Drawing for the job (mm, zero at the part's lowest x, y, z). Coordinates: 2 decimals unless noted, no trailing zeros. Write each loop counter-clockwise with the first axis right and the second up, starting at its lowest first coordinate (ties: lowest second). Pieces come first, ordered by that corner, then holes. Notation, with made-up numbers: M 55.5,32.5 L 112.5,32.5 A21 cw 112.5,37.5 Z; hole C -8,15 d7. An arc over 180 degrees is marked long. Put each result on its own line as item: value. Start each with the question number.
Q1. Cut at D-D (x = 14.75). Write the cut outline in (y, z), then the cut area to 3 significant figures.
Q2. Drill centre lines: line 1 along X through (y, z) = (2.75, 6.5); line 2 along X through (y, z) = (6.5, 6.5); line 3 along X through (y, z) = (4.75, 6.75). Where is each one in solid material? Low to high.
Q3. Cut at C-C (y = 5.25). Write the cut outline in (x, z).
Q4. Pull direction Z, two halves, no side cores. Call the marked faces 1, 2, 3 and 4: pulls with the +Z half, pulls with the -Z half, needs draft (parallel to the pull), parting line crosses it, or undercut.
Q5. Cut at B-B (z = 6.5). Write the cut outline in (x, y).
Q6. Cut at A-A (y = 7). Write the cut outline in (x, z).
Q7. Drop flat-ended pins along their axis: pin 1 (2 mm diameter, centred on y = 4, z = 11.5, fed in from +X); pin 2 (1.5 mm diameter, centred on y = 5.5, z = 10, fed in from -X). Give the stop position or say it passes through.
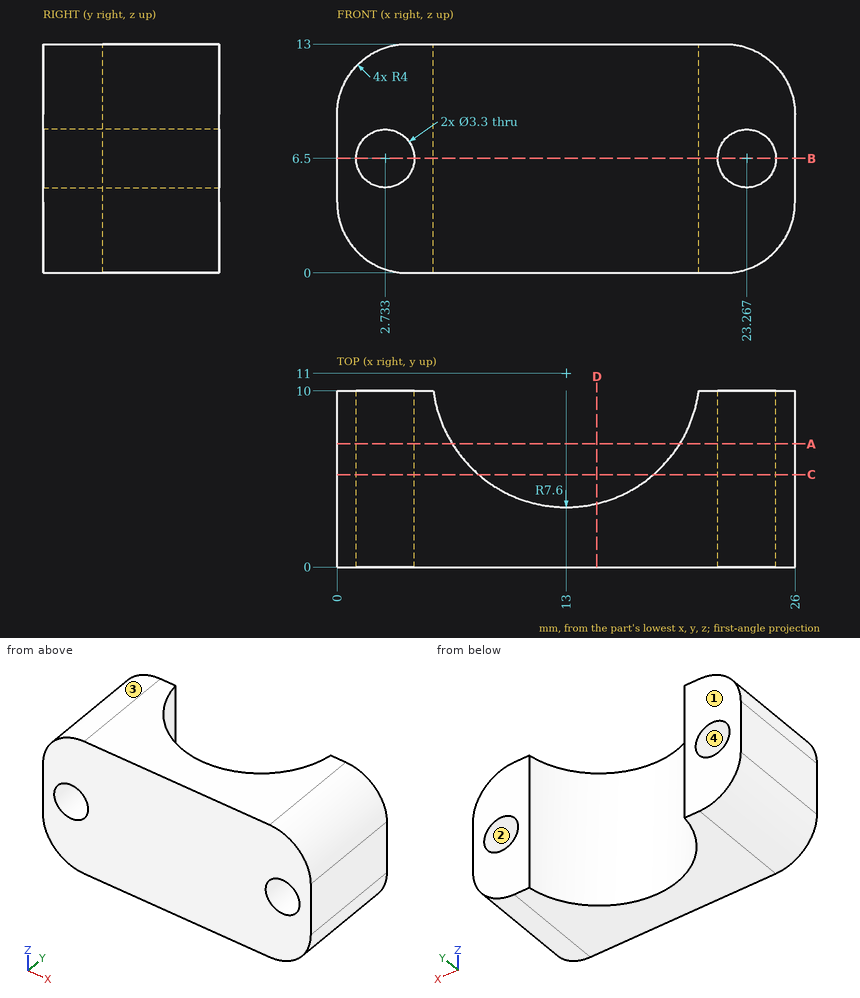
Computed values:
1. outline: M 0,0 L 3.6,0 L 3.6,13 L 0,13 Z
1. area: 46.9 mm2
2. line 1: 0 to 1.08, 4.38 to 21.62, 24.92 to 26
2. line 2: 0 to 1.08, 4.38 to 6.88, 19.12 to 21.62, 24.92 to 26
2. line 3: 0 to 1.1, 4.36 to 8.68, 17.32 to 21.64, 24.9 to 26
3. outline: M 0,4 A4 ccw 4,0 L 8.03,0 L 8.03,13 L 4,13 A4 ccw 0,9 Z; M 17.97,0 L 22,0 A4 ccw 26,4 L 26,9 A4 ccw 22,13 L 17.97,13 Z; hole C 2.73,6.5 d3.3; hole C 23.27,6.5 d3.3
4. face 1: needs draft
4. face 2: undercut
4. face 3: pulls with the +Z half
4. face 4: undercut
5. outline: M 0,0 L 1.08,0 L 1.08,10 L 0,10 Z; M 4.38,0 L 21.62,0 L 21.62,10 L 20.53,10 A7.6 cw 5.47,10 L 4.38,10 Z; M 24.92,0 L 26,0 L 26,10 L 24.92,10 Z
6. outline: M 0,4 A4 ccw 4,0 L 6.54,0 L 6.54,13 L 4,13 A4 ccw 0,9 Z; M 19.46,0 L 22,0 A4 ccw 26,4 L 26,9 A4 ccw 22,13 L 19.46,13 Z; hole C 2.73,6.5 d3.3; hole C 23.27,6.5 d3.3
7. pin 1: x = 25.71
7. pin 2: x = 0.01
